Answer from the drawing. Dimensions are ordinates in mm from the lowest x, y and z of the part. Coordinates: 2 decimals unless noted, no trailing zeros. Order: outer loops, then holes, each group sorted by start corner. A loop starts at its lowest first (then second) coordinate and runs counter-clockwise, first axis right, second up. Notation, with made-up numbers: (-16.75, -34) -> (12.25, -34) arc R21 ccw to (12.25, -8) -> close; hole circle Ø3 at (42, 8). An arc over 180 degrees is marked (long way). Answer in a Markdown table with one row per item.
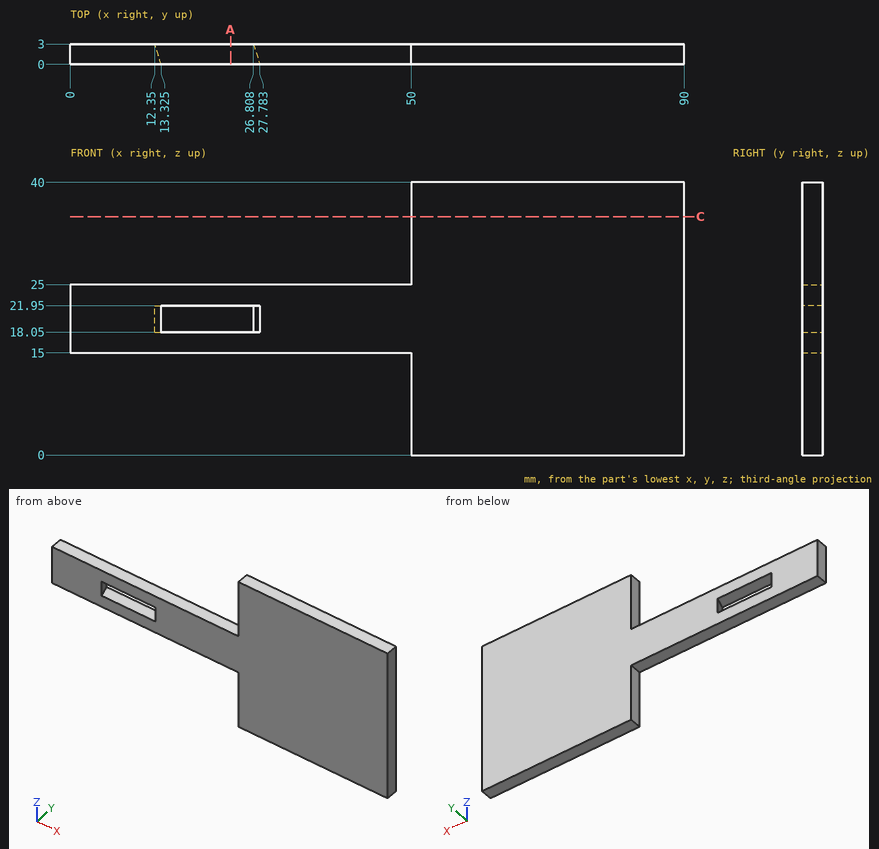
Q1. Consider line 1 (Z direction, x = 21.5, y = 0.8); line 2 (Z direction, x = 4, y = 2.55); line 3 (X direction, y = 0.6, z = 4). Determine where each line is inside the solid, lowest interval first.
Outcome:
| item | result |
|---|---|
| line 1 | 15 to 18.05, 21.95 to 25 |
| line 2 | 15 to 25 |
| line 3 | 50 to 90 |
Q2. The part is cut by section C-C (z = 35). Write down the section's boundary in (x, y).
Outcome:
| item | result |
|---|---|
| outline | (50, 0) -> (90, 0) -> (90, 3) -> (50, 3) -> close |
Q3. The part is cut by section A-A (x = 23.5). Write down the section's boundary in (y, z), then the cut area to 3 significant figures.
Outcome:
| item | result |
|---|---|
| outline | (0, 15) -> (3, 15) -> (3, 18.05) -> (0, 18.05) -> close; (0, 21.95) -> (3, 21.95) -> (3, 25) -> (0, 25) -> close |
| area | 18.3 mm² |
Q4. Given pin 1 (0.9 mm diameter, centred on x = 17, y = 2, fed in from +Z); pin 2 (12 mm diameter, centred on x = 62, z = 12, fed in from -Y); pin 3 (1 mm diameter, centred on x = 34, y = 0.5, fed in from -Z), each flat-ended and moving along its own axis, determine where each tip first touches the part or whether it passes through.
Outcome:
| item | result |
|---|---|
| pin 1 | z = 25 |
| pin 2 | y = 0 |
| pin 3 | z = 15 |
